Geometry check sheet. Reference: the model listing, model coordinates, mm. Face numbers are marked on the shaded views. A direction names the side the tool comes from. Give positions to 0.01 mm unless a question says otherwise; leave off trailing zeros. Loops run counter-clockwise (first coordinate to the right, second up) from the corner with the lowest first, then second, coordinate; pieces in that order, holes last.
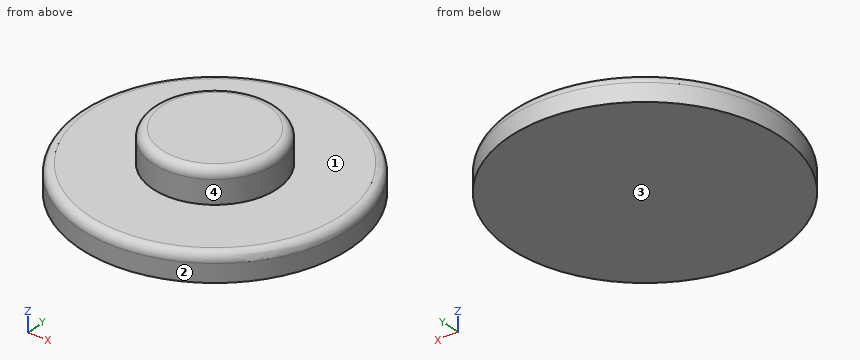
```python
from build123d import *

# Parameters (mm, degrees)
F0_R     = 7.5
F1_DEPTH = 1.5
F2_R     = 3.45
F3_DEPTH = 1.8
F4_R     = 0.5
F5_R     = 0.5


with BuildPart() as f1:
    # F0 (on Top) → F1 (new body)
    with BuildSketch(Plane.XY):
        Circle(F0_R)
    extrude(amount=F1_DEPTH)

    # F2 (on face) → F3 (join)
    with BuildSketch(Plane.XY.offset(1.5)):
        Circle(F2_R)
    extrude(amount=F3_DEPTH)

    # F4
    f4_edges = [f1.edges().sort_by_distance(p)[0] for p in [
        (-3.45, 0, 3.3),
    ]]
    fillet(f4_edges, radius=F4_R)

    # F5
    f5_edges = [f1.edges().sort_by_distance(p)[0] for p in [
        (-7.5, 0, 1.5),
    ]]
    fillet(f5_edges, radius=F5_R)


solid = f1.part
```
1) Sectioned sample at C-C on z = 2.4. Enter the section's corners in (x, y), plus the area to 3 significant figures.
2) Sectioned sample at D-D on z = 0.3. Enter the section's corners in (x, y).
3) Depth check by flat-ended pin: P1, Ø1.5, axis at x = 2, z = 2.5, coming from the +Y side; P2, Ø1.5, axis at y = -4, z = 2, coming from the +X side; P3, Ø5, axis at x = 0, y = 3.5, coming from the -Z side; P4, Ø1, axis at x = 5, z = 0.5, coming from the -Y side. Enter the tip coordinate at first touch or a pass-through.
4) Sectioned sample at A-A on y = 0. Enter the section's corners in (x, z).
5) Tool access check on the marked faces 3 and 4. Record the directions out of +Z, -Z, +X, -X, +Y, -Y that give a thin tool (end or side, any length) a straight path to the whole face; none if there is none.
6) Mould release check, pull along X, two halves, no side actions. Record for the marked faces 1 and 2: +X half, -X half, draft (parallel to the pull), parting line (faces both ways), or undercut.
7) Scan lines: line 1 along Z through (x, y) = (-3.5, -0.25); line 2 along Z through (x, y) = (-0.25, 3); line 3 along X through (y, z) = (3.75, 1.3). Record each from-to range of solid material in increasing order.
Determined:
1. outline: circle Ø6.9 at (0, 0)
1. area: 37.4 mm2
2. outline: circle Ø15 at (0, 0)
3. P1: stops at y = 3.22
3. P2: stops at x = 6.4
3. P3: stops at z = 0
3. P4: stops at y = -6
4. outline: (-7.5, 0) - (7.5, 0) - (7.5, 1) arc R0.5 ccw to (7, 1.5) - (3.45, 1.5) - (3.45, 2.8) arc R0.5 ccw to (2.95, 3.3) - (-2.95, 3.3) arc R0.5 ccw to (-3.45, 2.8) - (-3.45, 1.5) - (-7, 1.5) arc R0.5 ccw to (-7.5, 1) - close
5. face 3: -Z, +X, -X, +Y, -Y
5. face 4: +Z
6. face 1: draft
6. face 2: parting line
7. line 1: z = 0 to 1.5
7. line 2: z = 0 to 3.3
7. line 3: x = -6.38 to 6.38
